```python
from build123d import *

# Parameters (mm, degrees)
F2_R         = 10
F3_DEPTH     = 30.001
F4_R         = 1
F5_T3_ANGLE  = 72.4183645551
F5_T6_ANGLE  = 34.3109861798
F5_T9_ANGLE  = 34.3109861798
F5_T12_ANGLE = 72.4183645551
F5_T15_ANGLE = 34.3109861798
F5_T18_ANGLE = 72.4183645551
F5_T21_ANGLE = 34.3109861799
F5_T24_ANGLE = 72.4183645551
F5_T27_ANGLE = 34.3109861798
F5_T30_ANGLE = 72.4183645551
F5_T33_ANGLE = 34.3109861799
F5_T36_ANGLE = 72.4183645551
F5_T39_ANGLE = 34.3109861799
F5_T42_ANGLE = 72.4183645551
F5_T45_ANGLE = 34.3109861799
F5_T48_ANGLE = 72.4183645551
F5_T51_ANGLE = 34.3109861798
F5_T54_ANGLE = 72.4183645551
F6_R         = 8.5
F7_DEPTH     = 10


# Not quite as in the source:
# - a fillet or chamfer that OpenCascade refuses, or shapes differently, is made with other operations: its cross-section is extruded or revolved along the edge and cut away or added


with BuildPart() as f1:
    # F0 (on Front) → F1 (revolve)
    with BuildSketch(Plane.XZ):
        Polygon((8, 8), (8.6999093082, 0), (18.6999093082, 0), (25, 5.2864037759), (25, 30), (19.25, 30), (16.25, 27), (16.25, 20), (8.5, 20), (8.5, 33.5), (7.5, 34.5), (3.2, 34.5), (3.2, 8), align=None)
    revolve(axis=Axis((0, 0, 15.2192509614), (0, 0, 1)))

    # F2 (on face) → F3 (cut, through all)
    with BuildSketch(Plane.XY.offset(30)):
        with Locations((11.6286848731, 31.9495491067)):
            Circle(F2_R)
        with Locations((-11.6286848731, 31.9495491067)):
            Circle(F2_R)
        with Locations((-29.4448637287, 17)):
            Circle(F2_R)
        with Locations((-33.4834636024, -5.9040380407)):
            Circle(F2_R)
        with Locations((-21.8547787293, -26.045511066)):
            Circle(F2_R)
        with Locations((0, -34)):
            Circle(F2_R)
        with Locations((21.8547787293, -26.045511066)):
            Circle(F2_R)
        with Locations((33.4834636024, -5.9040380407)):
            Circle(F2_R)
        with Locations((29.4448637287, 17)):
            Circle(F2_R)
    extrude(amount=-F3_DEPTH, mode=Mode.SUBTRACT)

    # F4
    f4_edges = [f1.edges().sort_by_distance(p)[0] for p in [
        (-8.699909, 0, 0),
        (-18.699909, 0, 0),
    ]]
    fillet(f4_edges, radius=F4_R)

    # F5: fillet of radius 1 on 18 edges, made by hand


with BuildPart() as f5_tool1:
    # F5_s2 → F5_t3 (revolve)
    with BuildSketch(Plane(origin=(4.7878159953, -19.5059893322, 0), x_dir=(0, 0, 1), z_dir=(0.2383778196, -0.971172495, 0))):
        with BuildLine():
            ThreePointArc((29, 17.4334321252), (29.7071067812, 17.1405389064), (30, 16.4334321252))
            Line((30, 16.4334321252), (30, 17.4334321252))
            Line((30, 17.4334321252), (29, 17.4334321252))
        make_face()
    revolve(axis=Axis((-21.8547787293, -26.045511066, 30), (0, 0, 1)), revolution_arc=F5_T3_ANGLE)


with BuildPart() as f5_tool4:
    # F5_s5 → F5_t6 (revolve)
    with BuildSketch(Plane(origin=(0, 0, 0), x_dir=(0, 0, 1), z_dir=(-0.7969993255, 0.6039801944, 0))):
        with BuildLine():
            ThreePointArc((29, -25), (29.7071067812, -24.7071067812), (30, -24))
            Line((30, -24), (30, -25))
            Line((30, -25), (29, -25))
        make_face()
    revolve(axis=Axis((0, 0, 30), (0, 0, 1)), revolution_arc=F5_T6_ANGLE)


with BuildPart() as f5_tool7:
    # F5_s8 → F5_t9 (revolve)
    with BuildSketch(Plane(origin=(0, 0, 0), x_dir=(0, 0, 1), z_dir=(-0.222305919, 0.974976963, 0))):
        with BuildLine():
            ThreePointArc((29, -25), (29.7071067812, -24.7071067812), (30, -24))
            Line((30, -24), (30, -25))
            Line((30, -25), (29, -25))
        make_face()
    revolve(axis=Axis((0, 0, 30), (0, 0, 1)), revolution_arc=F5_T9_ANGLE)


with BuildPart() as f5_tool10:
    # F5_s11 → F5_t12 (revolve)
    with BuildSketch(Plane(origin=(-8.8705284196, -18.0200035347, 0), x_dir=(0, 0, 1), z_dir=(-0.4416496426, -0.897187602, 0))):
        with BuildLine():
            ThreePointArc((29, 17.4334321252), (29.7071067812, 17.1405389064), (30, 16.4334321252))
            Line((30, 16.4334321252), (30, 17.4334321252))
            Line((30, 17.4334321252), (29, 17.4334321252))
        make_face()
    revolve(axis=Axis((-33.4834636024, -5.9040380407, 30), (0, 0, 1)), revolution_arc=F5_T12_ANGLE)


with BuildPart() as f5_tool13:
    # F5_s14 → F5_t15 (revolve)
    with BuildSketch(Plane(origin=(0, 0, 0), x_dir=(0, 0, 1), z_dir=(0.4564068976, 0.889771175, 0))):
        with BuildLine():
            ThreePointArc((29, -25), (29.7071067812, -24.7071067812), (30, -24))
            Line((30, -24), (30, -25))
            Line((30, -25), (29, -25))
        make_face()
    revolve(axis=Axis((0, 0, 30), (0, 0, 1)), revolution_arc=F5_T15_ANGLE)


with BuildPart() as f5_tool16:
    # F5_s17 → F5_t18 (revolve)
    with BuildSketch(Plane(origin=(-18.378254002, -8.1022578133, 0), x_dir=(0, 0, 1), z_dir=(-0.9150243287, -0.4033986588, 0))):
        with BuildLine():
            ThreePointArc((29, 17.4334321252), (29.7071067812, 17.1405389064), (30, 16.4334321252))
            Line((30, 16.4334321252), (30, 17.4334321252))
            Line((30, 17.4334321252), (29, 17.4334321252))
        make_face()
    revolve(axis=Axis((-29.4448637287, 17, 30), (0, 0, 1)), revolution_arc=F5_T18_ANGLE)


with BuildPart() as f5_tool19:
    # F5_s20 → F5_t21 (revolve)
    with BuildSketch(Plane(origin=(0, 0, 0), x_dir=(0, 0, 1), z_dir=(0.9215618544, 0.3882315655, 0))):
        with BuildLine():
            ThreePointArc((29, -25), (29.7071067812, -24.7071067812), (30, -24))
            Line((30, -24), (30, -25))
            Line((30, -25), (29, -25))
        make_face()
    revolve(axis=Axis((0, 0, 30), (0, 0, 1)), revolution_arc=F5_T21_ANGLE)


with BuildPart() as f5_tool22:
    # F5_s23 → F5_t24 (revolve)
    with BuildSketch(Plane(origin=(-19.2865902853, 5.6066243856, 0), x_dir=(0, 0, 1), z_dir=(-0.960248962, 0.2791450001, 0))):
        with BuildLine():
            ThreePointArc((29, 17.4334321252), (29.7071067812, 17.1405389064), (30, 16.4334321252))
            Line((30, 16.4334321252), (30, 17.4334321252))
            Line((30, 17.4334321252), (29, 17.4334321252))
        make_face()
    revolve(axis=Axis((-11.6286848731, 31.9495491067, 30), (0, 0, 1)), revolution_arc=F5_T24_ANGLE)


with BuildPart() as f5_tool25:
    # F5_s26 → F5_t27 (revolve)
    with BuildSketch(Plane(origin=(0, 0, 0), x_dir=(0, 0, 1), z_dir=(0.9555077776, -0.2949659082, 0))):
        with BuildLine():
            ThreePointArc((29, -25), (29.7071067812, -24.7071067812), (30, -24))
            Line((30, -24), (30, -25))
            Line((30, -25), (29, -25))
        make_face()
    revolve(axis=Axis((0, 0, 30), (0, 0, 1)), revolution_arc=F5_T27_ANGLE)


with BuildPart() as f5_tool28:
    # F5_s29 → F5_t30 (revolve)
    with BuildSketch(Plane(origin=(-11.1705166275, 16.6921047237, 0), x_dir=(0, 0, 1), z_dir=(-0.556162434, 0.8310736111, 0))):
        with BuildLine():
            ThreePointArc((29, 17.4334321252), (29.7071067812, 17.1405389064), (30, 16.4334321252))
            Line((30, 16.4334321252), (30, 17.4334321252))
            Line((30, 17.4334321252), (29, 17.4334321252))
        make_face()
    revolve(axis=Axis((11.6286848731, 31.9495491067, 30), (0, 0, 1)), revolution_arc=F5_T30_ANGLE)


with BuildPart() as f5_tool31:
    # F5_s32 → F5_t33 (revolve)
    with BuildSketch(Plane(origin=(0, 0, 0), x_dir=(0, 0, 1), z_dir=(0.5423609923, -0.8401455553, 0))):
        with BuildLine():
            ThreePointArc((29, -25), (29.7071067812, -24.7071067812), (30, -24))
            Line((30, -24), (30, -25))
            Line((30, -25), (29, -25))
        make_face()
    revolve(axis=Axis((0, 0, 30), (0, 0, 1)), revolution_arc=F5_T33_ANGLE)


with BuildPart() as f5_tool34:
    # F5_s35 → F5_t36 (revolve)
    with BuildSketch(Plane(origin=(2.1723659067, 19.9671637495, 0), x_dir=(0, 0, 1), z_dir=(0.1081586779, 0.9941336431, 0))):
        with BuildLine():
            ThreePointArc((29, 17.4334321252), (29.7071067812, 17.1405389064), (30, 16.4334321252))
            Line((30, 16.4334321252), (30, 17.4334321252))
            Line((30, 17.4334321252), (29, 17.4334321252))
        make_face()
    revolve(axis=Axis((29.4448637287, 17, 30), (0, 0, 1)), revolution_arc=F5_T36_ANGLE)


with BuildPart() as f5_tool37:
    # F5_s38 → F5_t39 (revolve)
    with BuildSketch(Plane(origin=(0, 0, 0), x_dir=(0, 0, 1), z_dir=(-0.4564068976, 0.889771175, 0))):
        with BuildLine():
            ThreePointArc((29, 25), (29.7071067812, 24.7071067812), (30, 24))
            Line((30, 24), (30, 25))
            Line((30, 25), (29, 25))
        make_face()
    revolve(axis=Axis((0, 0, 30), (0, 0, -1)), revolution_arc=F5_T39_ANGLE)


with BuildPart() as f5_tool40:
    # F5_s41 → F5_t42 (revolve)
    with BuildSketch(Plane(origin=(14.49877429, 13.8993649467, 0), x_dir=(0, 0, 1), z_dir=(0.7218711424, 0.692027495, 0))):
        with BuildLine():
            ThreePointArc((29, 17.4334321252), (29.7071067812, 17.1405389064), (30, 16.4334321252))
            Line((30, 16.4334321252), (30, 17.4334321252))
            Line((30, 17.4334321252), (29, 17.4334321252))
        make_face()
    revolve(axis=Axis((33.4834636024, -5.9040380407, 30), (0, 0, 1)), revolution_arc=F5_T42_ANGLE)


with BuildPart() as f5_tool43:
    # F5_s44 → F5_t45 (revolve)
    with BuildSketch(Plane(origin=(0, 0, 0), x_dir=(0, 0, 1), z_dir=(-0.7332018585, -0.6800110548, 0))):
        with BuildLine():
            ThreePointArc((29, -25), (29.7071067812, -24.7071067812), (30, -24))
            Line((30, -24), (30, -25))
            Line((30, -25), (29, -25))
        make_face()
    revolve(axis=Axis((0, 0, 30), (0, 0, 1)), revolution_arc=F5_T45_ANGLE)


with BuildPart() as f5_tool46:
    # F5_s47 → F5_t48 (revolve)
    with BuildSketch(Plane(origin=(20.0410450471, 1.327898811, 0), x_dir=(0, 0, 1), z_dir=(0.9978120766, 0.0661139909, 0))):
        with BuildLine():
            ThreePointArc((29, 17.4334321252), (29.7071067812, 17.1405389064), (30, 16.4334321252))
            Line((30, 16.4334321252), (30, 17.4334321252))
            Line((30, 17.4334321252), (29, 17.4334321252))
        make_face()
    revolve(axis=Axis((21.8547787293, -26.045511066, 30), (0, 0, 1)), revolution_arc=F5_T48_ANGLE)


with BuildPart() as f5_tool49:
    # F5_s50 → F5_t51 (revolve)
    with BuildSketch(Plane(origin=(0, 0, 0), x_dir=(0, 0, 1), z_dir=(-0.9987678899, -0.0496256197, 0))):
        with BuildLine():
            ThreePointArc((29, -25), (29.7071067812, -24.7071067812), (30, -24))
            Line((30, -24), (30, -25))
            Line((30, -25), (29, -25))
        make_face()
    revolve(axis=Axis((0, 0, 30), (0, 0, 1)), revolution_arc=F5_T51_ANGLE)


with BuildPart() as f5_tool52:
    # F5_s53 → F5_t54 (revolve)
    with BuildSketch(Plane(origin=(16.2058880953, -11.8649059363, 0), x_dir=(0, 0, 1), z_dir=(0.8068656507, -0.5907349843, 0))):
        with BuildLine():
            ThreePointArc((29, 17.4334321252), (29.7071067812, 17.1405389064), (30, 16.4334321252))
            Line((30, 16.4334321252), (30, 17.4334321252))
            Line((30, 17.4334321252), (29, 17.4334321252))
        make_face()
    revolve(axis=Axis((0, -34, 30), (0, 0, 1)), revolution_arc=F5_T54_ANGLE)


with BuildPart() as f1_1:
    add(f1.part)

    # F5_t55: cut F5_tool1, F5_tool4, F5_tool7, F5_tool10, F5_tool13, F5_tool16, F5_tool19, F5_tool22, F5_tool25, F5_tool28, F5_tool31, F5_tool34, F5_tool37, F5_tool40, F5_tool43, F5_tool46, F5_tool49, F5_tool52
    add([f5_tool1.part, f5_tool4.part, f5_tool7.part, f5_tool10.part, f5_tool13.part, f5_tool16.part, f5_tool19.part, f5_tool22.part, f5_tool25.part, f5_tool28.part, f5_tool31.part, f5_tool34.part, f5_tool37.part, f5_tool40.part, f5_tool43.part, f5_tool46.part, f5_tool49.part, f5_tool52.part], mode=Mode.SUBTRACT)

    # F6 (on face) → F7 (cut, through all)
    with BuildSketch(Plane.XY.offset(30)):
        Polygon((9.3819418743, 16.25), (-9.3819418743, 16.25), (-18.7638837487, 0), (-9.3819418743, -16.25), (9.3819418743, -16.25), (18.7638837487, 0), align=None)
        Circle(F6_R, mode=Mode.SUBTRACT)
    extrude(amount=-F7_DEPTH, mode=Mode.SUBTRACT)


solid = f1_1.part
```
The model under review builds one solid part; all positions refer to its coordinate system, in mm. A direction names the side the tool comes from. Round coordinates to 2 decimals unless told otherwise and drop trailing zeros. Order: outer loops, then holes, each group sorted by start corner. A loop starts at its lowest first (then second) coordinate and runs counter-clockwise, first axis right, second up.
Item 1: Add section A-A, the plane z = 26. State the section outline as (x, y) points, and give its area (3 significant figures).
Working result:
outline: (-24.99, -0.62) arc R10 cw to (-23.7, -7.96) arc R25 ccw to (-18.75, -16.54) arc R10 cw to (-13.03, -21.33) arc R25 ccw to (-3.73, -24.72) arc R10 cw to (3.73, -24.72) arc R25 ccw to (13.03, -21.33) arc R10 cw to (18.75, -16.54) arc R25 ccw to (23.7, -7.96) arc R10 cw to (24.99, -0.62) arc R25 ccw to (23.27, 9.13) arc R10 cw to (19.55, 15.59) arc R25 ccw to (11.96, 21.95) arc R10 cw to (4.95, 24.5) arc R25 ccw to (-4.95, 24.5) arc R10 cw to (-11.96, 21.95) arc R25 ccw to (-19.55, 15.59) arc R10 cw to (-23.27, 9.13) arc R25 ccw to start; circle Ø17 at (0, 0); hole (-18.76, 0) - (-9.38, -16.25) - (9.38, -16.25) - (18.76, 0) - (9.38, 16.25) - (-9.38, 16.25) - close; hole circle Ø6.4 at (0, 0)
area: 1,200 mm2
Item 2: For pin 1 (8 mm diameter, centred on x = 19, y = -2.5, fed in from +Z); pin 2 (6 mm diameter, centred on x = -12.5, z = 12.5, fed in from +Y); pin 3 (4 mm diameter, centred on x = 6, z = 21, fed in from +Y); pin 4 (6 mm diameter, centred on x = 0, y = 0, fed in from +Z), all flat-tipped, find the tip position at first contact; note any pin that passes through.
Working result:
pin 1: stops at z = 30
pin 2: stops at y = 22.18
pin 3: stops at y = 24.68
pin 4: passes through
Item 3: Draft analysis for pull direction X (two halves, no side actions). For faces 1 (the cylindrical face through (0, 25, 17)), 2 (the conical face through (-1.073, 8.175, 5.194)), 3 (the cylindrical face through (21.616, -12.56, 17.309)), state which applies: released by +X, released by -X, zero draft, split by the parting line, or undercut.
Working result:
face 1: split by the parting line
face 2: undercut
face 3: released by +X
Item 4: Add section C-C, the plane z = 11. State the section outline as (x, y) points, and give its area (3 significant figures).
Working result:
outline: (-24.99, -0.62) arc R10 cw to (-23.7, -7.96) arc R25 ccw to (-18.75, -16.54) arc R10 cw to (-13.03, -21.33) arc R25 ccw to (-3.73, -24.72) arc R10 cw to (3.73, -24.72) arc R25 ccw to (13.03, -21.33) arc R10 cw to (18.75, -16.54) arc R25 ccw to (23.7, -7.96) arc R10 cw to (24.99, -0.62) arc R25 ccw to (23.27, 9.13) arc R10 cw to (19.55, 15.59) arc R25 ccw to (11.96, 21.95) arc R10 cw to (4.95, 24.5) arc R25 ccw to (-4.95, 24.5) arc R10 cw to (-11.96, 21.95) arc R25 ccw to (-19.55, 15.59) arc R10 cw to (-23.27, 9.13) arc R25 ccw to start; hole circle Ø6.4 at (0, 0)
area: 1,890 mm2
Item 5: Machinability: for faces 4 (the flat face through (-14.14, -8.01, 23.77)), 5 (the cylindrical face through (0, -24, 17)), 6 (the flat face through (-3.4, 0.1, 8)), which of the approach directions +Z, -Z, +X, -X, +Y, -Y give a long, thin tool a straight path to every point of the face, cutting with its end or side? Answer none if there is none.
Working result:
face 4: +Z
face 5: +Z, -Z, -Y
face 6: -Z
Item 6: To check wall thickness, follow probe 1 along Y at (x, z) = (0, 23); probe 2 along X at (y, z) = (6.5, 21); probe 3 along Y at (x, z) = (0, 28). State the ranges of each line that lie inside material, in increasing order.
Working result:
probe 1: y = -24 to -16.25, -8.5 to -3.2, 3.2 to 8.5, 16.25 to 25
probe 2: x = -24.14 to -15.01, -5.48 to 5.48, 15.01 to 24.14
probe 3: y = -24 to -17.25, -8.5 to -3.2, 3.2 to 8.5, 17.25 to 25
